Print and shaded views of the part. All mm, measured from the part's lowest x, y and z. A direction names the side the tool comes from. Give positions to 0.01 mm unless a question says otherwise; leave off trailing zeros. Write each loop counter-clockwise with the first axis right and the second up, starting at its lowest first coordinate (ties: lowest second). Pieces come first, ordered by that corner, then holes. Notation, with made-up numbers: (-27, 25) -> (-6, 25) arc R18 cw to (-6, 58) -> close; hole circle Ø10 at (16, 36). An arc over 180 degrees is marked (long way). Put each result on its own line as item: value.
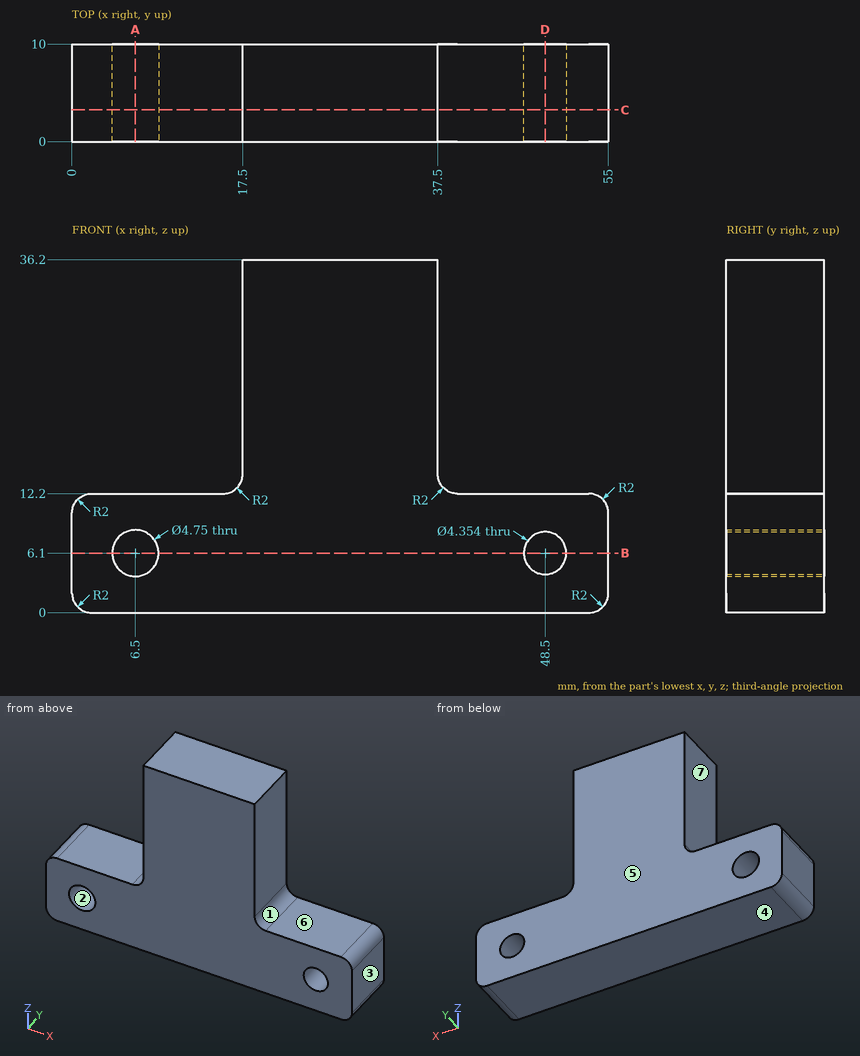
1) Slice it at A-A (x = 6.5). Write the cut outline in (y, z) (1 decimal).
Filled sheet:
outline: (0, 0) -> (10, 0) -> (10, 3.7) -> (0, 3.7) -> close; (0, 8.5) -> (10, 8.5) -> (10, 12.2) -> (0, 12.2) -> close
2) Pin check, flat tips, straight feed: pin 1 (3 mm diameter, centred on y = 6.5, z = 22, fed in from +X); pin 2 (3 mm diameter, centred on y = 8.5, z = 14, fed in from +X) (1 decimal); pin 3 (3 mm diameter, centred on x = 43.5, y = 3.5, fed in from +Z). Stop position of each tip, or through.
Filled sheet:
pin 1: x = 37.5
pin 2: x = 38.4
pin 3: z = 12.2
3) Tool access for the marked faces 5, 6 and 7: list every direction of +Z, -Z, +X, -X, +Y, -Y with a clear straight run to the whole face (end or side of a thin tool).
Filled sheet:
face 5: +Z, -Z, +X, -X, +Y
face 6: +Z, +X, +Y, -Y
face 7: +Z, -X, +Y, -Y
4) Slice it at C-C (y = 3.25). Give the number of separate pieces and of enclosed holes in the cut face, plus the area to 3 significant figures.
Filled sheet:
separate pieces: 1
enclosed holes: 2
area: 1,120 mm2
5) Slice it at D-D (x = 48.5). Write the cut outline in (y, z).
Filled sheet:
outline: (0, 0) -> (10, 0) -> (10, 3.92) -> (0, 3.92) -> close; (0, 8.28) -> (10, 8.28) -> (10, 12.2) -> (0, 12.2) -> close
6) Pull direction Z, two halves, no side cores. Call the marked faces 1, 2, 3 and 4: released by +Z, released by -Z, zero draft, split by the parting line, or undercut.
Filled sheet:
face 1: released by +Z
face 2: undercut
face 3: zero draft
face 4: released by -Z
7) Slice it at B-B (z = 6.1). Write the cut outline in (x, y) (1 decimal), plus the area to 3 significant figures.
Filled sheet:
outline: (0, 0) -> (4.1, 0) -> (4.1, 10) -> (0, 10) -> close; (8.9, 0) -> (46.3, 0) -> (46.3, 10) -> (8.9, 10) -> close; (50.7, 0) -> (55, 0) -> (55, 10) -> (50.7, 10) -> close
area: 459 mm2
8) Wall check: L1, parallel to Z at x = 48.5, y = 7; L2, parallel to Z at x = 6.5, y = 3.75 (1 decimal); L3, parallel to X at y = 1.25, z = 27.5. Give the ranges that are in metal, low to high.
Filled sheet:
L1: 0 to 3.92, 8.28 to 12.2
L2: 0 to 3.7, 8.5 to 12.2
L3: 17.5 to 37.5
